Geometry check sheet. Reference: the model listing, model coordinates, mm. Face numbers are marked on the shaded views. Round coordinates to 2 decimals unless told otherwise and drop trailing zeros. Write each loop counter-clockwise with the first axis right and the second up, starting at its lowest first coordinate (ties: lowest second). Pieces come first, ordered by that corner, then holes. Notation, with made-up numbers: (-37.5, 66.5) -> (5.5, 66.5) arc R15 ccw to (5.5, 93.5) -> close; hole circle Ø9 at (88, 85.25). An arc over 180 degrees is marked (long way). Return JSON: item names as keys, results as strings. Group by question number.
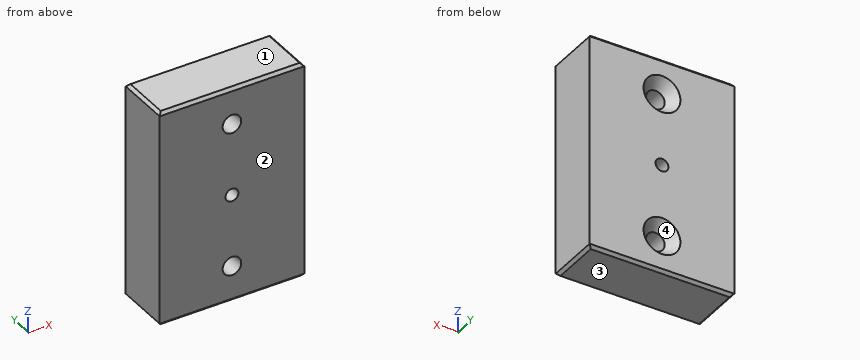
from build123d import *

# Parameters (mm, degrees)
SKETCH1_W                                         = 25.4
SKETCH1_H                                         = 9.525
BOSS_EXTRUDE1_DEPTH                               = 38.1
CSK_FOR_4_FLAT_HEAD_SOCKET_CAP_SCREW1_D           = 3.2639
CSK_FOR_4_FLAT_HEAD_SOCKET_CAP_SCREW1_DEPTH       = 9.525
CSK_FOR_4_FLAT_HEAD_SOCKET_CAP_SCREW1_CSINK_D     = 6.477
CSK_FOR_4_FLAT_HEAD_SOCKET_CAP_SCREW1_CSINK_ANGLE = 82
F_4_40_TAPPED_HOLE1_D                             = 2.2606
F_4_40_TAPPED_HOLE1_DEPTH                         = 9.525
CHAMFER1_SIZE                                     = 0.508


with BuildPart() as part:
    # Sketch1 → Boss-Extrude1 (new body)
    with BuildSketch(Plane.XY):
        Rectangle(SKETCH1_W, SKETCH1_H)
    extrude(amount=BOSS_EXTRUDE1_DEPTH)

    # CSK for #4 Flat Head Socket Cap Screw1
    with Locations(Plane(origin=(0, 4.7625, 0), x_dir=(1, 0, 0), z_dir=(0, 1, 0))):
        with Locations((0, -6.35), (0, -31.75)):
            CounterSinkHole(CSK_FOR_4_FLAT_HEAD_SOCKET_CAP_SCREW1_D / 2, CSK_FOR_4_FLAT_HEAD_SOCKET_CAP_SCREW1_CSINK_D / 2, depth=CSK_FOR_4_FLAT_HEAD_SOCKET_CAP_SCREW1_DEPTH, counter_sink_angle=CSK_FOR_4_FLAT_HEAD_SOCKET_CAP_SCREW1_CSINK_ANGLE)

    # #4-40 Tapped Hole1
    with Locations(Plane(origin=(0, 4.7625, 0), x_dir=(1, 0, 0), z_dir=(0, 1, 0))):
        with Locations((0, -19.05)):
            Hole(F_4_40_TAPPED_HOLE1_D / 2, depth=F_4_40_TAPPED_HOLE1_DEPTH)

    # Chamfer1
    chamfer1_edges = [part.edges().sort_by_distance(p)[0] for p in [
        (12.7, 0, 38.1),
        (0, 4.7625, 38.1),
        (-12.7, 0, 38.1),
        (0, 4.7625, 0),
        (12.7, 0, 0),
        (0, -4.7625, 0),
        (-12.7, 0, 0),
        (0, -4.7625, 38.1),
    ]]
    chamfer(chamfer1_edges, length=CHAMFER1_SIZE)


solid = part.part
1) Sectioned sample at B-B on z = 31.75. Enter the section's corners in (x, y), and give its area (3 significant figures).
2) Sectioned sample at C-C on y = -2.5. Enter the section's corners in (x, z).
3) Go/stop test with flat-tipped pins: P1, Ø5, axis at x = 0, z = 6.35, coming from the +Y side; P2, Ø4, axis at x = 0, z = 31.75, coming from the +Y side; P3, Ø2.5, axis at x = 0, z = 19.05, coming from the +Y side. Record where each tip stops, or that it passes through.
4) Material ranges on probe 1 along Z at (x, y) = (0, -1.5); probe 2 along X at (y, z) = (-1.5, 6.35); probe 3 along Z at (x, y) = (-0.5, 2), recorded low to high. Write a range as [from, to].
5) Mould release check, pull along Z, two halves, no side actions. Record for the marked faces 1, 2, 3 and 4: +Z half, -Z half, draft (parallel to the pull), parting line (faces both ways), or undercut.
6) Sectioned sample at A-A on x = 0. Enter the section's corners in (y, z).
Evaluation:
{
 "1": {"outline": "(-12.7, -4.76) -> (-1.63, -4.76) -> (-1.63, 2.91) -> (-3.24, 4.76) -> (-12.7, 4.76) -> close; (1.63, -4.76) -> (12.7, -4.76) -> (12.7, 4.76) -> (3.24, 4.76) -> (1.63, 2.91) -> close", "area": "208 mm2"},
 "2": {"outline": "(-12.7, 0.51) -> (-12.19, 0) -> (12.19, 0) -> (12.7, 0.51) -> (12.7, 37.59) -> (12.19, 38.1) -> (-12.19, 38.1) -> (-12.7, 37.59) -> close; hole circle Ø3.26 at (0, 6.35); hole circle Ø3.26 at (0, 31.75); hole circle Ø2.26 at (0, 19.05)"},
 "3": {"P1": "stops at y = 3.91", "P2": "stops at y = 3.34", "P3": "stops at y = 4.76"},
 "4": {"probe 1": "z = [0, 4.72], [7.98, 17.92], [20.18, 30.12], [33.38, 38.1]", "probe 2": "x = [-12.7, -1.63], [1.63, 12.7]", "probe 3": "z = [0, 4.8], [7.9, 18.04], [20.06, 30.2], [33.3, 38.1]"},
 "5": {"face 1": "+Z half", "face 2": "draft", "face 3": "-Z half", "face 4": "undercut"},
 "6": {"outline": "(-4.76, 0.51) -> (-4.25, 0) -> (4.25, 0) -> (4.76, 0.51) -> (4.76, 3.11) -> (2.91, 4.72) -> (-4.76, 4.72) -> close; (-4.76, 7.98) -> (2.91, 7.98) -> (4.76, 9.59) -> (4.76, 17.92) -> (-4.76, 17.92) -> close; (-4.76, 20.18) -> (4.76, 20.18) -> (4.76, 28.51) -> (2.91, 30.12) -> (-4.76, 30.12) -> close; (-4.76, 33.38) -> (2.91, 33.38) -> (4.76, 34.99) -> (4.76, 37.59) -> (4.25, 38.1) -> (-4.25, 38.1) -> (-4.76, 37.59) -> close"}
}
